Autodesk Inventor part; units mm, degrees
ref_plane "YZ Plane" through (0, 0, 0) normal (1, 0, 0) x (0, 1, 0)
ref_plane "XZ Plane" through (0, 0, 0) normal (0, 1, 0) x (-1, 0, 0)
ref_plane "XY Plane" through (0, 0, 0) normal (0, 0, 1) x (1, 0, 0)
sketch "Sketch7" plane through (0, 0, 0) normal (0, 0, 1) x (1, 0, 0)
  line L0 (0, 0) -> (0, 20)
  line L1 (-20, 0) -> (0, 0)
  line L2 (-20, 8) -> (-8, 8)
  line L3 (-8, 8) -> (-8, 20)
  line L4 (-8, 8) -> (0, 0)
  line L5 (0, 20) -> (-8, 20)
  line L6 (-20, 0) -> (-20, 8)
  dimension "d40" = 20
  dimension "d43" = 45
  dimension "d44" = 8
extrude "Extrusion4" add sketch "Sketch7" along normal mid plane 40
sketch "Sketch8" plane through (-8, 8, 20) normal (-1, 0, 0) x (0, 0, 1)
  line L0 (-31, 2) -> (-9, 2) construction
  line L1 (-40, -8) -> (0, -8)
  point P0 (-20, -8)
  point P1 (-20, 2)
  point P2 (-20, -8)
  dimension "d45" = 10
  dimension "d53" = 22
hole "Hole3" at (-8, 10, -11) at (-8, 10, 11) direction (1, 0, 0) diameter 5.8 end through all
sketch "Sketch9" plane through (-20, 0, 20) normal (0, -1, 0) x (1, 0, 0)
  line L0 (20, 0) -> (20, -40)
  point P0 (20, -20)
  point P1 (10, -20)
  point P2 (20, -20)
  point P3 (20, -20)
  dimension "d54" = 10
hole "Hole4" at (-10, 0, 0) direction (0, 1, 0) diameter 5.8 end through all
sketch "Sketch10" plane through (0, 0, 0) normal (0, 0, 1) x (1, 0, 0)
  line L0 (0, 20) -> (0, 0)
  line L1 (0, 0) -> (-20, 0)
  line L2 (-20, 0) -> (-20, 20)
  line L3 (-20, 20) -> (0, 20)
  line L4 (0, 20) -> (0, 0)
  line L5 (0, 0) -> (-20, 0)
  line L6 (-20, 0) -> (-20, 8)
  line L7 (-20, 8) -> (-8, 8)
  line L8 (-8, 8) -> (-8, 20)
  line L9 (-8, 20) -> (0, 20)
extrude "Extrusion5" add sketch "Sketch10" along normal mid plane 40 contours L8 L7 L2 L3
sketch "Sketch11" plane through (-10, 8, 0) normal (0, -1, 0) x (0, 0, 1)
  circle A0 centre (0, 0) radius 2.9
  point P0 (0, -10)
  point P1 (0, 0)
hole "Hole5" at (-10, 8, 0) direction (0, 1, 0) diameter 11 end through all
sketch "Sketch12" plane through (-8, 10, 11) normal (1, 0, 0) x (0, 0, -1)
  circle A0 centre (22, 0) radius 2.9
  circle A1 centre (0, 0) radius 2.9
  point P0 (11, -10)
hole "Hole6" at (-8, 10, -11) at (-8, 10, 11) direction (-1, 0, 0) diameter 11 end through all
fillet "Fillet4" radius 2 4 edges at (0, 10, 20) (-20, 10, 20) (0, 10, -20) (-20, 10, -20)
chamfer "Chamfer3" distance 0.6 angle 45 14 edges at (-20, 20, 0) (-10, 20, 20) (-0.5858, 20, 19.4142) (0, 20, 0) (-0.5858, 20, -19.4142) (-10, 20, -20) (-20, 0, 0) (-19.4142, 0, 19.4142) (-10, 0, 20) (-0.5858, 0, 19.4142) (0, 0, 0) (-0.5858, 0, -19.4142) (-10, 0, -20) (-19.4142, 0, -19.4142)
chamfer "Chamfer4" distance 0.6 angle 45 1 edges at (-10, 0, 2.9)
move or copy body "Move Body1" bodies to move or copy 1 copy no rotation origin (0, 0, 0) rotation axis (1, 0, 0) rotation angle 90
properties part number "2020-perp-connecdtor"
The model under review builds one solid part; all positions refer to its coordinate system, in mm. A direction names the side the tool comes from. Round coordinates to 2 decimals unless told otherwise and drop trailing zeros. Loops run counter-clockwise (first coordinate to the right, second up) from the corner with the lowest first, then second, coordinate; pieces in that order, holes last. Notation, with made-up numbers: (-24, 84) -> (29, 84) arc R8 cw to (29, 92) -> close; hole circle Ø10 at (2.5, -7). An arc over 180 degrees is marked (long way). Answer as a JSON object with one key per item and string values. Group by question number.
1) For pin 1 Ø3.5 at (y, z) = (11, 10) entering from -X; pin 2 Ø3.5 at (x, y) = (-8, 1) entering from +Z; pin 3 Ø9 at (y, z) = (-10.5, 9.5) entering from -X, all flat-tipped, find the tip position at first contact; note any pin that passes through.
2) We need section B-B on z = 11.5. Write out the cut boundary in (x, y), then the cut area to 3 significant figures.
3) We need section C-C on x = -2.75. Write out the cut boundary in (y, z), then the cut area to 3 significant figures.
4) For line 1 (Y direction, x = -16.25, z = 9.75); line 2 (Z direction, x = -17.25, y = 11); line 3 (Y direction, x = -16, z = 5.5), list the stretches that pass through material, from the lowest coordinate up. Write a range as [from, to].
5) We need section D-D on z = 5.5. Write out the cut boundary in (x, y), then the cut area to 3 significant figures.
6) Mouldability with a two-part tool opening along Z and no side actions: class faces 1 (the face through (-7.6, 2.4, 8)), 2 (the face through (-8, -8.6, 12.4)), 3 (the face through (-20, 0, 10)) as released by +Z, released by -Z, zero draft, split by the parting line, or undercut.
7) For faces 4 (the face through (-0.83, -19.15, 19.76)), 5 (the face through (-4.63, -1.19, 14.08)), 6 (the face through (-14.1, 13.5, 14.9)), list the 3-axis set-ups (+Z, -Z, +X, -X, +Y, -Y) from which the entire face can be reached by the end or side of a thin tool; tool diameter is ignored.
8) We need section A-A on y = 11. Write out the cut boundary in (x, z), then the cut area to 3 significant figures.
Result set:
{
 "1": {"pin 1": "through", "pin 2": "z = 8", "pin 3": "x = -8"},
 "2": {"outline": "(-20, -18) arc R2 ccw to (-18, -20) -> (-2, -20) arc R2 ccw to (0, -18) -> (0, -13.48) -> (-8, -13.48) -> (-8, -16.29) -> (-20, -16.29) -> close; (-20, -5.71) -> (-8, -5.71) -> (-8, -8.52) -> (0, -8.52) -> (0, 8.52) -> (-8, 8.52) -> (-8, 5.71) -> (-20, 5.71) -> close; (-20, 16.29) -> (-8, 16.29) -> (-8, 13.48) -> (0, 13.48) -> (0, 18) arc R2 ccw to (-2, 20) -> (-18, 20) arc R2 ccw to (-20, 18) -> close; hole circle Ø11 at (-10, 0)", "area": "368 mm²"},
 "3": {"outline": "(-20, 0.6) -> (-19.4, 0) -> (19.4, 0) -> (20, 0.6) -> (20, 19.4) -> (19.4, 20) -> (-19.4, 20) -> (-20, 19.4) -> close; hole circle Ø5.8 at (-11, 10); hole circle Ø5.8 at (11, 10)", "area": "746 mm²"},
 "4": {"line 1": "[-20, -16.49], [-5.51, 5.51], [16.49, 20]", "line 2": "[0, 4.5], [15.5, 20]", "line 3": "[-20, -14.16], [-7.84, 7.84], [14.16, 20]"},
 "5": {"outline": "(-20, -18) arc R2 ccw to (-18, -20) -> (-2, -20) arc R2 ccw to (0, -18) -> (0, 18) arc R2 ccw to (-2, 20) -> (-18, 20) arc R2 ccw to (-20, 18) -> (-20, 14.16) -> (-8, 14.16) -> (-8, 7.84) -> (-20, 7.84) -> (-20, -7.84) -> (-8, -7.84) -> (-8, -14.16) -> (-20, -14.16) -> close; hole circle Ø5.8 at (-10, 0)", "area": "618 mm²"},
 "6": {"face 1": "released by +Z", "face 2": "undercut", "face 3": "zero draft"},
 "7": {"face 4": "+Z, +X, -Y", "face 5": "+Z", "face 6": "-X"},
 "8": {"outline": "(-20, 0.6) -> (-19.4, 0) -> (-0.6, 0) -> (0, 0.6) -> (0, 7.1) -> (-8, 7.1) -> (-8, 4.5) -> (-20, 4.5) -> close; (-20, 15.5) -> (-8, 15.5) -> (-8, 12.9) -> (0, 12.9) -> (0, 19.4) -> (-0.6, 20) -> (-19.4, 20) -> (-20, 19.4) -> close", "area": "221 mm²"}
}
